Geometry check sheet. Reference: the model listing, model coordinates, mm. Face numbers are marked on the shaded views. A direction names the side the tool comes from. Give positions to 0.01 mm unless a question says otherwise; leave off trailing zeros. Write each loop counter-clockwise with the first axis right and the second up, starting at its lowest first coordinate (ties: lowest second). Pieces come first, ordered by that corner, then holes. Notation, with made-up numbers: (51, -0.5) - (55, -0.5) arc R22 cw to (55, 19.5) - close; hole circle Ø10 at (70, 38). An arc over 180 degrees is marked (long way). Write item = value, one per line. Start each with the question number.
(1) Draft check along X on the marked faces 3, 4 and 5. Enter one of: pulls with the +X half, pulls with the -X half, needs draft (parallel to the pull), parting line crosses it, or undercut.
(2) Access from +Z, -Z, +X, -X, +Y, -Y to the whole of each face (thin tool, end or side, straight path). Record for the marked faces 1 and 2.
(3) Depth check by flat-ended pin: pin 1 Ø1.5 at (y, z) = (11.5, 5.5) entering from +X; pin 2 Ø1.5 at (y, z) = (-2, 3) entering from +X; pin 3 Ø3 at (x, z) = (-20, 11) entering from -Y. Enter the tip coordinate at first touch or a pass-through.
(4) Section check B-B, the plane x = 16. Enter the section's corners in (y, z), plus the area to 3 significant figures.
(5) Thickness scan on L1, parallel to X at y = 0.5, z = 6; L2, parallel to X at y = -0.5, z = 2.5; L3, parallel to X at y = 13.25, z = 3.25. Record the ranges inside material, lowest first.
(6) Section check C-C, the plane y = 2.75. Give the number of separate pieces and of enclosed holes in the cut face, plus the area to 3 significant figures.
(7) Section check A-A, the plane z = 7.5. Enter the section's corners in (x, y).
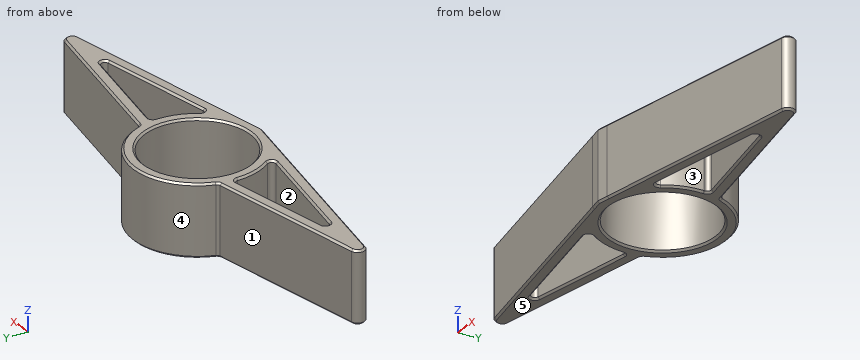
```python
from build123d import *

# Parameters (mm, degrees)
F0_R     = 11.1
F1_DEPTH = 15
F2_R     = 0.8
F3_R     = 1.5
F4_SIZE  = 0.4


with BuildPart() as f1:
    # F0 (on Top) → F1 (new body)
    with BuildSketch(Plane.XY):
        with BuildLine():
            Line((-12.915164, 7.651788), (-55, 0))
            Line((-55, 0), (-2.414954, -9.560917))
            ThreePointArc((-2.414954, -9.560917), (-6.417434, -8.155817), (-9.786299, -5.578047))
            Line((-9.786299, -5.578047), (-40.465558, 0))
            Line((-40.465558, 0), (-13.447354, 4.912401))
            ThreePointArc((-13.447354, 4.912401), (-13.252232, 6.295883), (-12.915164, 7.651788))
        make_face()
        with BuildLine():
            ThreePointArc((12.915164, 7.651788), (0, 17.221326), (-12.915164, 7.651788))
            ThreePointArc((-12.915164, 7.651788), (-13.252232, 6.295883), (-13.447354, 4.912401))
            ThreePointArc((-13.447354, 4.912401), (-12.746099, -0.726927), (-9.786299, -5.578047))
            ThreePointArc((-9.786299, -5.578047), (-6.417434, -8.155817), (-2.414954, -9.560917))
            ThreePointArc((-2.414954, -9.560917), (0, -9.778674), (2.414954, -9.560917))
            ThreePointArc((2.414954, -9.560917), (6.417434, -8.155817), (9.786299, -5.578047))
            ThreePointArc((9.786299, -5.578047), (12.537245, -1.285417), (13.5, 3.721326))
            ThreePointArc((13.5, 3.721326), (13.486832, 4.317445), (13.447354, 4.912401))
            ThreePointArc((13.447354, 4.912401), (13.252232, 6.295883), (12.915164, 7.651788))
        make_face()
        with Locations((0, 3.721326)):
            Circle(F0_R, mode=Mode.SUBTRACT)
        with BuildLine():
            ThreePointArc((2.414954, -9.560917), (0, -9.778674), (-2.414954, -9.560917))
            Line((-2.414954, -9.560917), (0, -10))
            Line((0, -10), (2.414954, -9.560917))
        make_face()
        with BuildLine():
            Line((55, 0), (12.915164, 7.651788))
            ThreePointArc((12.915164, 7.651788), (13.252232, 6.295883), (13.447354, 4.912401))
            Line((13.447354, 4.912401), (40.465558, 0))
            Line((40.465558, 0), (9.786299, -5.578047))
            ThreePointArc((9.786299, -5.578047), (6.417434, -8.155817), (2.414954, -9.560917))
            Line((2.414954, -9.560917), (55, 0))
        make_face()
    extrude(amount=F1_DEPTH)

    # F2
    f2_edges = [f1.edges().sort_by_distance(p)[0] for p in [
        (-40.465558, 0, 7.5),
        (40.465558, 0, 7.5),
        (-9.786299, -5.578047, 7.5),
        (9.786299, -5.578047, 7.5),
        (-13.447354, 4.912401, 7.5),
        (13.447354, 4.912401, 7.5),
        (12.915164, 7.651788, 7.5),
        (-12.915164, 7.651788, 7.5),
    ]]
    fillet(f2_edges, radius=F2_R)

    # F3
    f3_edges = [f1.edges().sort_by_distance(p)[0] for p in [
        (55, 0, 7.5),
        (-55, 0, 7.5),
    ]]
    fillet(f3_edges, radius=F3_R)

    # F4
    f4_edges = [f1.edges().sort_by_distance(p)[0] for p in [
        (-30.134502, 4.521, 15),
        (-48.114745, 0, 15),
        (-13.007334, 7.746806, 15),
        (-23.441537, -5.737902, 15),
        (0, 17.221326, 15),
        (23.441537, -5.737902, 15),
        (13.007334, 7.746806, 15),
        (48.114745, 0, 15),
        (30.134502, 4.521, 15),
        (-11.1, 3.721326, 15),
        (12.919215, -0.195801, 15),
        (13.78088, 4.554757, 15),
        (11.094527, -4.838669, 15),
        (25.288948, 2.759384, 15),
        (24.023167, -2.989526, 15),
        (36.793422, 0, 15),
        (-24.023167, -2.989526, 15),
        (-11.094527, -4.838669, 15),
        (-36.793422, 0, 15),
        (-12.919215, -0.195801, 15),
        (-25.288948, 2.759384, 15),
        (-13.78088, 4.554757, 15),
        (-30.134502, 4.521, 0),
        (-48.114745, 0, 0),
        (-13.007334, 7.746806, 0),
        (-23.441537, -5.737902, 0),
        (0, 17.221326, 0),
        (23.441537, -5.737902, 0),
        (13.007334, 7.746806, 0),
        (48.114745, 0, 0),
        (30.134502, 4.521, 0),
        (-11.1, 3.721326, 0),
        (12.919215, -0.195801, 0),
        (11.094527, -4.838669, 0),
        (13.78088, 4.554757, 0),
        (24.023167, -2.989526, 0),
        (25.288948, 2.759384, 0),
        (36.793422, 0, 0),
        (-24.023167, -2.989526, 0),
        (-11.094527, -4.838669, 0),
        (-36.793422, 0, 0),
        (-12.919215, -0.195801, 0),
        (-25.288948, 2.759384, 0),
        (-13.78088, 4.554757, 0),
    ]]
    chamfer(f4_edges, length=F4_SIZE)


solid = f1.part
```
Model answer:
q1.face_3 = undercut
q1.face_4 = parting line crosses it
q1.face_5 = needs draft
q2.face_1 = +Z, -Z, -X, +Y
q2.face_2 = +Z, -Z
q3.pin_1 = 11.53
q3.pin_2 = 47.44
q3.pin_3 = -6.64
q4.outline = (-7.09, 0.4) - (-6.68, 0) - (-4.85, 0) - (-4.45, 0.4) - (-4.45, 14.6) - (-4.85, 15) - (-6.68, 15) - (-7.09, 14.6) - close; (4.45, 0.4) - (4.85, 0) - (6.68, 0) - (7.09, 0.4) - (7.09, 14.6) - (6.68, 15) - (4.85, 15) - (4.45, 14.6) - close
q4.area = 78.6 mm²
q5.L1 = -48.03 to -36.62, -13.11 to -10.62, 10.62 to 13.11, 36.62 to 48.03
q5.L2 = -48.03 to -36.62, -12.82 to -10.27, 10.27 to 12.82, 36.62 to 48.03
q5.L3 = -9.56 to -5.69, 5.69 to 9.56
q6.separate_pieces = 4
q6.enclosed_holes = 0
q6.area = 504 mm²
q7.outline = (-46.88, -1.48) - (-2.41, -9.56) - (0, -10) - (2.41, -9.56) - (46.88, -1.48) arc R1.5 ccw to (46.88, 1.48) - (13.39, 7.57) arc R0.8 cw to (12.77, 8.09) arc R13.5 ccw to (-12.77, 8.09) arc R0.8 cw to (-13.39, 7.57) - (-46.88, 1.48) arc R1.5 ccw to start; hole (-36.14, -0.79) - (-11.91, -5.19) arc R0.8 ccw to (-11.11, -3.95) arc R13.5 cw to (-13.5, 3.93) arc R0.8 ccw to (-14.44, 4.73) - (-36.14, 0.79) arc R0.8 ccw to start; hole circle Ø22.2 at (0, 3.72); hole (11.11, -3.95) arc R0.8 ccw to (11.91, -5.19) - (36.14, -0.79) arc R0.8 ccw to (36.14, 0.79) - (14.44, 4.73) arc R0.8 ccw to (13.5, 3.93) arc R13.5 cw to (13.5, 3.72) arc R13.5 cw to start
